Autodesk Inventor part; units mm, degrees
ref_plane "YZ Plane" through (0, 0, 0) normal (1, 0, 0) x (0, 1, 0)
ref_plane "XZ Plane" through (0, 0, 0) normal (0, 1, 0) x (-1, 0, 0)
ref_plane "XY Plane" through (0, 0, 0) normal (0, 0, 1) x (1, 0, 0)
sketch "Sketch1" plane through (0, 0, 0) normal (0, 1, 0) x (-1, 0, 0)
  circle A0 centre (0, 0) radius 2.44
  circle A1 centre (0, 0) radius 4.2
  line L0 (1.1547, -2) -> (-1.1547, -2)
  line L1 (-1.1547, -2) -> (-2.3094, 0)
  line L2 (-2.3094, 0) -> (-1.1547, 2)
  line L3 (-1.1547, 2) -> (1.1547, 2)
  line L4 (1.1547, 2) -> (2.3094, 0)
  line L5 (2.3094, 0) -> (1.1547, -2)
  dimension "d0" = 4.88
  dimension "d1" = 8.4
  dimension "d8" = 4
extrude "Extrusion1" add sketch "Sketch1" along normal blind 5 contours A0 | A1 | L0 L1 L2 L3 L4 L5
extrude "Extrusion2" add sketch "Sketch1" against normal blind 40 contours A0 | L0 L1 L2 L3 L4 L5
extrude "Extrusion3" cut sketch "Sketch1" against normal blind 3 from surface at 5 contours L0 L1 L2 L3 L4 L5
fillet "Fillet1" radius 0.5 1 edges at (4.2, 5, 0)
thread "Thread2"
equation "\"d4\" = length"
equation "\"length\" = 40"
properties part number "M5x20"
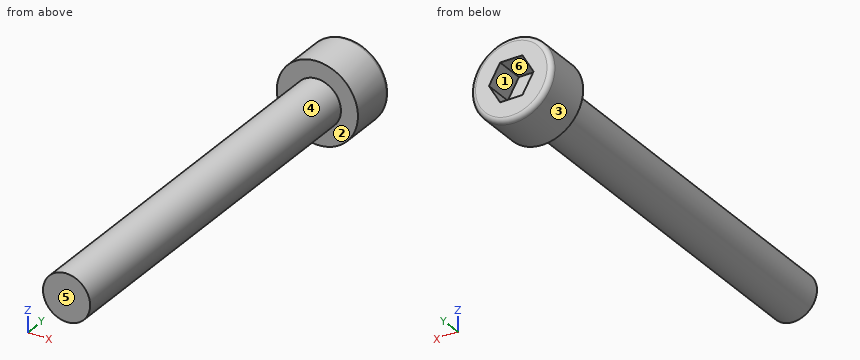
Check sheet for the modelled part. Datum: model origin and axes. Units: mm. Face numbers are marked on the shaded views. A direction names the side the tool comes from. Coordinates: 2 decimals unless noted, no trailing zeros. Loops run counter-clockwise (first coordinate to the right, second up) from the corner with the lowest first, then second, coordinate; pieces in that order, holes last. Notation, with made-up numbers: M 65.25,87.5 L 111.25,87.5 A33 ccw 111.25,124.5 Z; hole C 28,6.5 d5. An arc over 180 degrees is marked long. Answer as a JSON object with one key per item and string values.
1. Sectioned sample at B-B on y = -24. Record the cut outline in (x, z), and give its area (3 significant figures).
Outcome:
{"outline": "C 0,0 d4.88", "area": "18.7 mm²"}
2. Release check for a two-part mould opening along X. For the marked faces 1, 2 and 3 record: pulls with the +X half, pulls with the -X half, needs draft (parallel to the pull), parting line crosses it, or undercut.
Outcome:
{"face 1": "undercut", "face 2": "needs draft", "face 3": "parting line crosses it"}
3. Sectioned sample at A-A on x = 0. Record the cut outline in (y, z), and give its area (3 significant figures).
Outcome:
{"outline": "M -40,-2.44 L 0,-2.44 L 0,-4.2 L 4.5,-4.2 A0.5 ccw 5,-3.7 L 5,-2 L 2,-2 L 2,2 L 5,2 L 5,3.7 A0.5 ccw 4.5,4.2 L 0,4.2 L 0,2.44 L -40,2.44 Z", "area": "225 mm²"}
4. Access from +Z, -Z, +X, -X, +Y, -Y to the whole of each face (thin tool, end or side, straight path). Record for the marked faces 4, 5 and 6.
Outcome:
{"face 4": "-Y", "face 5": "+Z, -Z, +X, -X, -Y", "face 6": "+Y"}
5. Depth check by flat-ended pin: P1, Ø2, axis at y = -4.5, z = -1.5, coming from the -X side; P2, Ø1.2, axis at x = -0.5, y = 4, coming from the -Z side; P3, Ø5, axis at x = -0.5, y = -5.5, coming from the -Z side; P4, Ø5, axis at x = 3.5, y = -3.5, coming from the -Z side. Enter the tip coordinate at first touch or a pass-through.
Outcome:
{"P1": "x = -2.39", "P2": "z = -4.2", "P3": "z = -2.44", "P4": "z = -2.23"}
6. Scan lines: L1, parallel to Y at x = -1.25, z = -3.25; L2, parallel to X at y = 0.5, z = -0.25; L3, parallel to Y at x = 1.5, z = 1. Record each from-to range of solid material in increasing order. Write a range as from..to.
Outcome:
{"L1": "0..5", "L2": "-4.19..4.19", "L3": "-40..2"}
